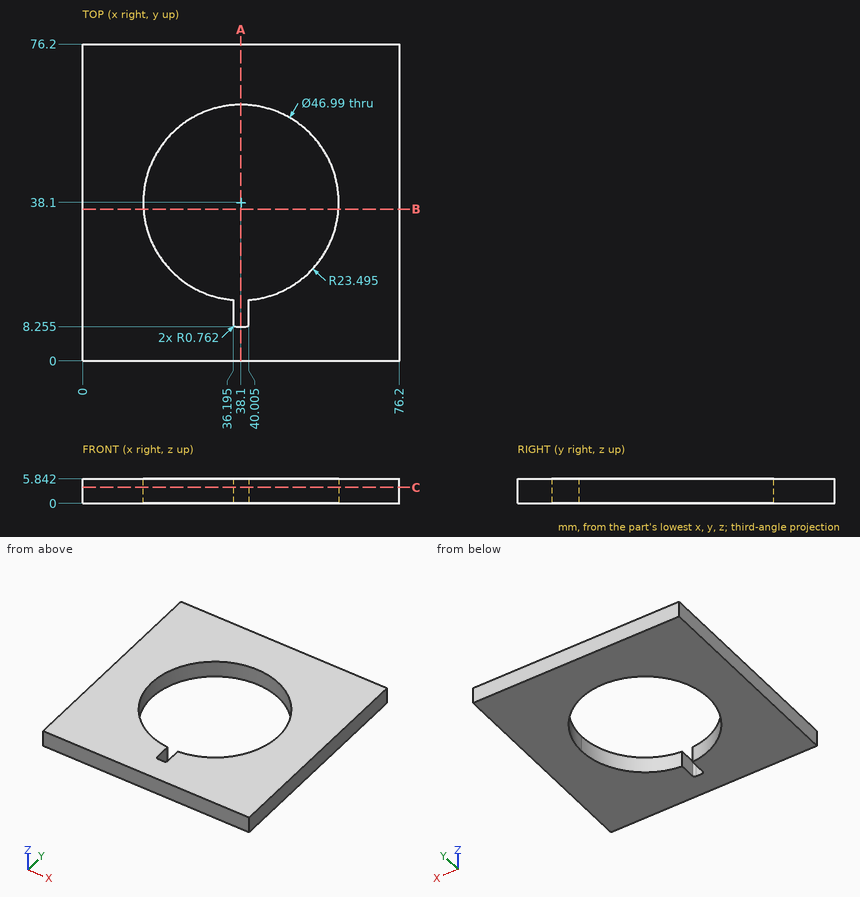
Input: dimensioned drawing with shaded views. Units: mm. Origin: part minimum x, y, z. Coordinates: 2 decimals unless noted, no trailing zeros. Write each loop counter-clockwise with the first axis right and the second up, starting at its lowest first coordinate (ties: lowest second). Pieces come first, ordered by that corner, then holes. Notation, with made-up numbers: M 34,52.5 L 59,52.5 A30 ccw 59,89.5 Z; hole C -25.5,-38.5 d7. An arc over 180 degrees is marked long. Use a Markdown table: item, result.
1) Section C-C, the plane z = 3.8. Output: boundary loops of the cut face in (x, y) (3 decimals).
Conclusion:
| item | result |
|---|---|
| outline | M 0,0 L 76.2,0 L 76.2,76.2 L 0,76.2 Z; hole M 36.195,9.017 A0.762 ccw 36.957,8.255 L 39.243,8.255 A0.762 ccw 40.005,9.017 L 40.005,14.682 A23.495 ccw long 36.195,14.682 Z |
2) Ray query, L1, parallel to Y at x = 38.1, z = 3.4 (3 decimals); L2, parallel to X at y = 38.1, z = 2.6 (3 decimals); L3, parallel to X at y = 14.5, z = 5.3 (3 decimals). Return the intervals inside material, ascending.
Conclusion:
| item | result |
|---|---|
| L1 | y = 0 to 8.255, 61.595 to 76.2 |
| L2 | x = 0 to 14.605, 61.595 to 76.2 |
| L3 | x = 0 to 36.195, 40.005 to 76.2 |
3) Section B-B, the plane y = 36.5. Output: boundary loops of the cut face in (x, z), then the cut area to 3 significant figures.
Conclusion:
| item | result |
|---|---|
| outline | M 0,0 L 14.66,0 L 14.66,5.84 L 0,5.84 Z; M 61.54,0 L 76.2,0 L 76.2,5.84 L 61.54,5.84 Z |
| area | 171 mm^2 |
4) Section A-A, the plane x = 38.1. Output: boundary loops of the cut face in (y, z) (3 decimals), then the cut area to 3 significant figures.
Conclusion:
| item | result |
|---|---|
| outline | M 0,0 L 8.255,0 L 8.255,5.842 L 0,5.842 Z; M 61.595,0 L 76.2,0 L 76.2,5.842 L 61.595,5.842 Z |
| area | 134 mm^2 |
